Input: part model. Units: mm. Frame: model coordinates. Round coordinates to 2 decimals unless told otherwise and drop trailing zeros. Loops run counter-clockwise (first coordinate to the right, second up) from the corner with the lowest first, then second, coordinate; pieces in that order, holes last. Notation, with made-up numbers: (59, 56) - (87, 56) arc R35 cw to (87, 95) - close; hole circle Ø2 at (33.25, 31). An arc over 180 degrees is marked (long way). One line per question, with ' | ' between items. Start each with the question number.
from build123d import *

# Parameters (mm, degrees)
SKETCH1_W                    = 1346.2
SKETCH1_H                    = 673.1
BOSS_EXTRUDE1_DEPTH          = 17.78
F_1_8_0_125_DIAMETER_HOLE1_D = 3.175
SKETCH4_W                    = 127
SKETCH4_H                    = 133.35
CUT_EXTRUDE1_DEPTH           = 753.758687031
SKETCH5_W                    = 1244.6
SKETCH5_H                    = 635
CUT_EXTRUDE2_DEPTH           = 9.525
FILLET1_R                    = 6.35


with BuildPart() as part:
    # Sketch1 → Boss-Extrude1 (new body)
    with BuildSketch(Plane(origin=(0, 0, 0), x_dir=(1, 0, 0), z_dir=(0, 1, 0))):
        Rectangle(SKETCH1_W, SKETCH1_H)
    extrude(amount=BOSS_EXTRUDE1_DEPTH)

    # 1/8 (0.125) Diameter Hole1 (through all)
    with Locations(Plane(origin=(0, 17.78, 0), x_dir=(1, 0, 0), z_dir=(0, 1, 0))):
        with Locations((0, 0), (457.2, 152.4), (-457.2, -152.4), (-457.2, 152.4), (457.2, -152.4)):
            Hole(F_1_8_0_125_DIAMETER_HOLE1_D / 2)

    # Sketch4 → Cut-Extrude1 (cut, through all)
    with BuildSketch(Plane(origin=(0, 17.78, 0), x_dir=(1, 0, 0), z_dir=(0, 1, 0))):
        with Locations((-609.6, 0)):
            Rectangle(SKETCH4_W, SKETCH4_H)
    extrude(amount=-CUT_EXTRUDE1_DEPTH, mode=Mode.SUBTRACT)

    # Sketch5 → Cut-Extrude2 (cut)
    with BuildSketch(Plane(origin=(0, 17.78, 0), x_dir=(1, 0, 0), z_dir=(0, 1, 0))):
        with Locations((-31.75, 0)):
            Rectangle(SKETCH5_W, SKETCH5_H)
    extrude(amount=-CUT_EXTRUDE2_DEPTH, mode=Mode.SUBTRACT)

    # Fillet1
    fillet1_edges = [part.edges().sort_by_distance(p)[0] for p in [
        (-673.1, 8.89, 66.675),
        (-673.1, 8.89, -66.675),
        (-546.1, 4.1275, -66.675),
        (-546.1, 4.1275, 66.675),
        (-654.05, 13.0175, 66.675),
        (-654.05, 13.0175, -66.675),
        (-654.05, 13.0175, 317.5),
        (590.55, 13.0175, -317.5),
        (673.1, 8.89, 336.55),
        (590.55, 13.0175, 317.5),
        (-673.1, 8.89, 336.55),
        (-654.05, 13.0175, -317.5),
        (-673.1, 8.89, -336.55),
        (673.1, 8.89, -336.55),
    ]]
    fillet(fillet1_edges, radius=FILLET1_R)


solid = part.part
(1) Line query: line 1 along Z through (x, y) = (-457.2, 3); line 2 along X through (y, z) = (4.25, -152.4); line 3 along X through (y, z) = (13.5, -229.5). Output: solid intervals per line, ascending. Write a range as from..to.
(2) Pin query (flat end, axial travel): P1, Ø3, axis at y = 10.5, z = -31.5, coming from the -X side; P2, Ø4, axis at x = -457.2, z = -152.4, coming from the +Y side (3 decimals); P3, Ø1.9, axis at x = 457.2, z = -152.4, coming from the -Y side; P4, Ø6.5, axis at y = 6, z = 24, coming from the -X side. Return the tip coordinate at first contact, or that it passes through.
(3) Section A-A, the plane z = -226.5. Output: boundary loops of the cut face in (x, y) (3 decimals).
(4) Section B-B, the plane y = 4.5. Give the number of separate pieces and of enclosed holes in the cut face, plus the area to 3 significant figures.
(5) Section C-C, the plane x = 118. Output: boundary loops of the cut face in (y, z) (3 decimals), plus the area to 3 significant figures.
(6) Pull-direction query (Z, two-part tool) for faces 1 (the face through (595, 17.78, -2)), 2 (the face through (-44, 8.255, -4)); classes: released by +Z, released by -Z, zero draft, split by the parting line, or undercut.
Derived:
1) line 1: z = -336.55..-153.99, -150.81..150.81, 153.99..336.55 | line 2: x = -673.1..-458.79, -455.61..455.61, 458.79..673.1 | line 3: x = -673.1..-654.05, 590.55..673.1
2) P1: stops at x = 590.55 | P2: stops at y = 8.255 | P3: passes through | P4: stops at x = -546.1
3) outline: (-673.1, 0) - (673.1, 0) - (673.1, 17.78) - (590.55, 17.78) - (590.55, 8.255) - (-654.05, 8.255) - (-654.05, 17.78) - (-673.1, 17.78) - close
4) separate pieces: 1 | enclosed holes: 5 | area: 889,000 mm²
5) outline: (0, -336.55) - (17.78, -336.55) - (17.78, -317.5) - (8.255, -317.5) - (8.255, 317.5) - (17.78, 317.5) - (17.78, 336.55) - (0, 336.55) - close | area: 5,920 mm²
6) face 1: zero draft | face 2: undercut
